Can you work these out from the model? Positions are in its coordinate system, mm. Face numbers are marked on the shaded views. Round coordinates to 2 decimals unless told otherwise and drop trailing zeros. Loops run counter-clockwise (first coordinate to the right, second up) from the corner with the lowest first, then second, coordinate; pieces in that order, holes last. Notation, with made-up numbers: (5, 30) - (42, 30) arc R12 ccw to (42, 49) - close; hole circle Ø6 at (60.5, -38). An arc over 180 degrees is marked (long way). Answer as CSV lines item,"result".
Autodesk Inventor part; units mm, degrees
ref_plane "Plan de construction1" through (0, 49.5, 0) normal (0, 1, 0) x (1, 0, 0)
ref_plane "Plan de construction2" through (0, 48, 0) normal (0, 1, 0) x (1, 0, 0)
ref_plane "YZ Plane" through (0, 0, 0) normal (1, 0, 0) x (0, 1, 0)
sketch "Esquisse1" plane through (0, 0, 0) normal (0, 1, 0) x (-1, 0, 0)
  line L0 (0, 0) -> (30, 0)
  line L1 (30, 0) -> (30, -30)
  line L2 (30, -30) -> (0, -30)
  line L3 (0, -30) -> (0, 0)
  line L4 (28, 0) -> (0, 0)
  line L5 (0, 0) -> (0, -198)
  line L6 (28, 0) -> (2, 0)
  line L7 (2, 0) -> (2, -28)
  line L8 (2, -28) -> (28, -28)
  line L9 (28, -28) -> (28, 0)
  dimension "d0" = 30
  dimension "d1" = 30
  dimension "d4" = 2
  dimension "d5" = 2
  dimension "d6" = 2
extrude "Extrusion1" add sketch "Esquisse1" along normal blind 50 contours L0 L7 L8 L9 L1 L2 L3
sketch "Esquisse2" plane through (0, 50, 0) normal (0, 1, 0) x (1, 0, 0)
  point P0 (0, 0)
  point P1 (-28, 0)
  point P2 (-2, 28)
ref_plane "Plan de construction1" through (0, 49.5, 0) normal (0, 1, 0) x (1, 0, 0)
ref_plane "Plan de construction2" through (0, 48, 0) normal (0, 1, 0) x (1, 0, 0)
sketch "Esquisse3" plane through (0, 49.5, 0) normal (0, 1, 0) x (1, 0, 0)
  line L0 (-28, 0) -> (-2, 0)
  line L1 (-2, 0) -> (-2, 28)
  line L2 (-2, 28) -> (-28, 28)
  line L3 (-28, 28) -> (-28, 0)
  line L4 (-27, 0) -> (-3, 0)
  line L5 (-3, 0) -> (-3, 27)
  line L6 (-3, 27) -> (-27, 27)
  line L7 (-27, 27) -> (-27, 0)
  point P0 (0, 0)
  dimension "d14" = 27
  dimension "d15" = 1
  dimension "d16" = 1
  dimension "d17" = 1
extrude "Extrusion2" add sketch "Esquisse3" along normal blind 0.5 contours L3 L2 L1 L0 L5 L6 L7
sketch "Esquisse4" plane through (0, 48, 0) normal (0, 1, 0) x (1, 0, 0)
  line L0 (-27, 0) -> (-3, 0)
  line L1 (-3, 0) -> (-3, 27)
  line L2 (-3, 27) -> (-27, 27)
  line L3 (-27, 27) -> (-27, 0)
  line L4 (-28, 0) -> (-2, 0)
  line L5 (-2, 0) -> (-2, 28)
  line L6 (-2, 28) -> (-28, 28)
  line L7 (-28, 28) -> (-28, 0)
  point P0 (0, 0)
extrude "Extrusion3" add sketch "Esquisse4" along normal blind 0.5 contours L4 L7 L6 L5 L1 L2 L3
properties part number "Pièce carré"
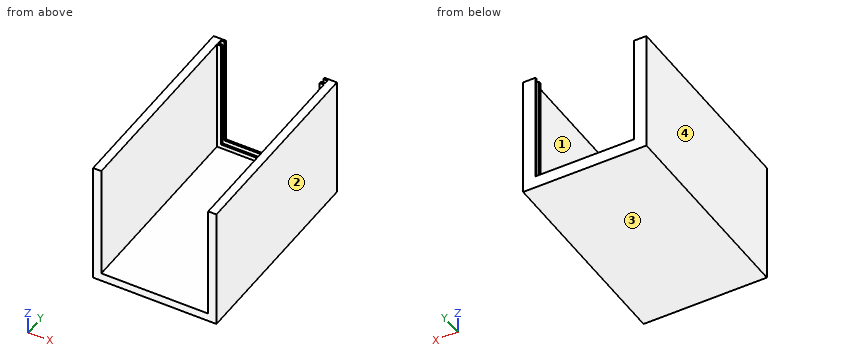
Q1. Imagine slicing it at A-A (z = -10). Write out the boundary of the cut face in (x, y).
Checks:
outline,"(-30, 0) - (-28, 0) - (-28, 48) - (-27, 48) - (-27, 48.5) - (-28, 48.5) - (-28, 49.5) - (-27, 49.5) - (-27, 50) - (-30, 50) - close; (-3, 48) - (-2, 48) - (-2, 0) - (0, 0) - (0, 50) - (-3, 50) - (-3, 49.5) - (-2, 49.5) - (-2, 48.5) - (-3, 48.5) - close"
Q2. We'd pull the mould along X, two halves only. Please class the marked faces 1, 2, 3 and 4: pulls with the +X half, pulls with the -X half, needs draft (parallel to the pull), parting line crosses it, or undercut.
Checks:
face 1,"undercut"
face 2,"pulls with the +X half"
face 3,"needs draft"
face 4,"pulls with the -X half"
Q3. If I drill on line 1 along X through (y, z) = (6.5, -26.25); line 2 along Z through (x, y) = (-14, 2), over which ranges is the centre line in solid material (lowest first)? Write a range as [from, to].
Checks:
line 1,"[-30, -28], [-2, 0]"
line 2,"[-30, -28]"
Q4. Imagine slicing it at B-B (x = -14.5). Write out the boundary of the cut face in (y, z), then the cut area to 3 significant figures.
Checks:
outline,"(0, -30) - (50, -30) - (50, -27) - (49.5, -27) - (49.5, -28) - (48.5, -28) - (48.5, -27) - (48, -27) - (48, -28) - (0, -28) - close"
area,"101 mm²"
Q5. I'm going to push flat-ended pins straight in: pin 1 Ø13 at (x, z) = (-12, -14) entering from -Y; pin 2 Ø3 at (x, y) = (-8.5, 20.5) entering from +Z; pin 3 Ø0.8 at (y, z) = (49, -9) entering from +X. Where does each tip first touch, or does it pass through?
Checks:
pin 1,"through"
pin 2,"z = -28"
pin 3,"x = 0"
Q6. Imagine slicing it at C-C (y = 15). Write out the boundary of the cut face in (x, z).
Checks:
outline,"(-30, -30) - (0, -30) - (0, 0) - (-2, 0) - (-2, -28) - (-28, -28) - (-28, 0) - (-30, 0) - close"
